Geometry: final body of the model. Coordinates: model frame, mm. Face numbers are marked on the shaded views. A direction names the side the tool comes from. Round coordinates to 2 decimals unless told otherwise and drop trailing zeros. Write each loop counter-clockwise with the first axis right and the second up, starting at its lowest first coordinate (ties: lowest second). Pieces come first, ordered by that corner, then holes. Notation, with made-up numbers: M 10,79.5 L 63,79.5 A21 ccw 63,98.5 Z; hole C 19.5,-1 d7. An arc over 180 degrees is marked long. Use one line per item in the form item = value. Start each with the question number.
Item 1: Pull-direction query (X, two-part tool) for the marked faces 1, 2 and 3; classes: pulls with the +X half, pulls with the -X half, needs draft (parallel to the pull), parting line crosses it, or undercut.
Item 2: Ray query, probe 1 along Y at (x, z) = (9, 0); probe 2 along Z at (x, y) = (0, 14); probe 3 along Y at (x, z) = (-1, 0). Return the intervals inside material, ascending.
Item 3: Section query C-C (z = 0). Return loops of the section in (x, y).
Item 4: Section query B-B (x = 0). Return loops of the section in (y, z), and give its area (3 significant figures).
Item 5: Reachability of the marked faces 4 and 5 from +Z, -Z, +X, -X, +Y, -Y: full face, straight path, thin tool, end or side. Return the list, or none.
Item 6: Section query D-D (y = 22). Return loops of the section in (x, z).
Item 7: Pin query (flat end, axial travel): pin 1 Ø1 at (x, y) = (1.5, 54.5) entering from -Z; pin 2 Ø2 at (y, z) = (11.5, 14) entering from +X; pin 3 Ø6 at (y, z) = (52.5, -1.5) entering from -X. Return the tip coordinate at first contact, or that it passes through.
Item 8: Section query A-A (y = 70). Return loops of the section in (x, z).
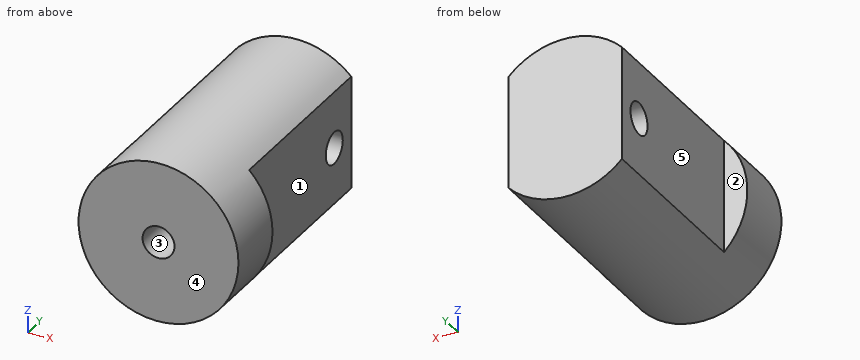
from build123d import *

# Parameters (mm, degrees)
SKETCH1_R           = 25
BOSS_EXTRUDE1_DEPTH = 80
CUT_EXTRUDE1_DEPTH  = 60
SKETCH3_R           = 5
CUT_EXTRUDE2_DEPTH  = 60
SKETCH4_R           = 5
CUT_EXTRUDE3_DEPTH  = 30


with BuildPart() as part:
    # Sketch1 → Boss-Extrude1 (new body)
    with BuildSketch(Plane(origin=(0, 0, 0), x_dir=(1, 0, 0), z_dir=(0, 1, 0))):
        Circle(SKETCH1_R)
    extrude(amount=BOSS_EXTRUDE1_DEPTH)

    # Sketch2 → Cut-Extrude1 (cut)
    with BuildSketch(Plane(origin=(0, 80, 0), x_dir=(1, 0, 0), z_dir=(0, 1, 0))):
        with BuildLine():
            Line((-17.708192822, -17.647093443), (-17.708192822, 17.647093443))
            ThreePointArc((-17.708192822, 17.647093443), (-25, 0), (-17.708192822, -17.647093443))
        make_face()
        with BuildLine():
            ThreePointArc((25, 0), (23.10524638, 9.547124684), (17.708192822, 17.647093443))
            Line((17.708192822, 17.647093443), (17.708192822, -17.647093443))
            ThreePointArc((17.708192822, -17.647093443), (23.10524638, -9.547124684), (25, 0))
        make_face()
    extrude(amount=-CUT_EXTRUDE1_DEPTH, mode=Mode.SUBTRACT)

    # Sketch3 → Cut-Extrude2 (cut)
    with BuildSketch(Plane(origin=(17.708192822, 0, 0), x_dir=(0, 0, -1), z_dir=(1, 0, 0))):
        with Locations((0, 70)):
            Circle(SKETCH3_R)
    extrude(amount=-CUT_EXTRUDE2_DEPTH, mode=Mode.SUBTRACT)

    # Sketch4 → Cut-Extrude3 (cut)
    with BuildSketch(Plane.XZ):
        Circle(SKETCH4_R)
    extrude(amount=-CUT_EXTRUDE3_DEPTH, mode=Mode.SUBTRACT)


solid = part.part
Working result:
q1.face_1 = pulls with the +X half
q1.face_2 = needs draft
q1.face_3 = undercut
q2.probe_1 = 0 to 65, 75 to 80
q2.probe_2 = -25 to -5, 5 to 25
q2.probe_3 = 30 to 65, 75 to 80
q3.outline = M -25,0 L -5,0 L -5,30 L 5,30 L 5,0 L 25,0 L 25,20 L 17.71,20 L 17.71,65 L -17.71,65 L -17.71,20 L -25,20 Z; M -17.71,75 L 17.71,75 L 17.71,80 L -17.71,80 Z
q4.outline = M 0,-25 L 80,-25 L 80,25 L 0,25 L 0,5 L 30,5 L 30,-5 L 0,-5 Z; hole C 70,0 d10
q4.area = 3,620 mm²
q5.face_4 = +Z, -Z, +X, -X, -Y
q5.face_5 = +Z, -Z, -X, +Y
q6.outline = M -17.71,-17.65 A25 ccw 17.71,-17.65 L 17.71,17.65 A25 ccw -17.71,17.65 Z; hole C 0,0 d10
q7.pin_1 = -24.98
q7.pin_2 = 21.35
q7.pin_3 = -17.71
q8.outline = M -17.71,-17.65 A25 ccw 17.71,-17.65 L 17.71,-5 L -17.71,-5 Z; M -17.71,5 L 17.71,5 L 17.71,17.65 A25 ccw -17.71,17.65 Z
